from build123d import *

# Parameters (mm, degrees)
F0_W     = 64
F0_H     = 10
F0_R     = 1.75
F1_DEPTH = 4
F2_R     = 2
F3_DEPTH = 10
F4_W     = 64
F4_H     = 9
F5_DEPTH = 6
F6_R     = 1.75
F7_DEPTH = 25
F8_W     = 6
F8_H     = 6
F9_DEPTH = 4
F10_R    = 2


with BuildPart() as f1:
    # F0 (on Front) → F1 (new body)
    with BuildSketch(Plane.XZ):
        Rectangle(F0_W, F0_H)
        with Locations((-27, 0)):
            Circle(F0_R, mode=Mode.SUBTRACT)
        with BuildLine():
            ThreePointArc((28.75, 0), (27, -1.75), (25.25, 0))
            ThreePointArc((25.25, 0), (27, 1.75), (28.75, 0))
        make_face(mode=Mode.SUBTRACT)
    extrude(amount=F1_DEPTH)

    # F2
    f2_edges = [f1.edges().sort_by_distance(p)[0] for p in [
        (-32, -2, 5),
        (32, -2, 5),
    ]]
    fillet(f2_edges, radius=F2_R)

    # F3 (add): a face of the model
    f3_faces = [f1.faces().sort_by_distance(p)[0] for p in [
        (0, -2, -5),
    ]]
    extrude(f3_faces, amount=F3_DEPTH)

    # F4 (on face) → F5 (join)
    with BuildSketch(Plane(origin=(0, 0, 0), x_dir=(-1, 0, 0), z_dir=(0, 1, 0))):
        with Locations((0, -10.5)):
            Rectangle(F4_W, F4_H)
    extrude(amount=F5_DEPTH)

    # F6 (on face) → F7 (cut)
    with BuildSketch(Plane(origin=(0, 6, 0), x_dir=(-1, 0, 0), z_dir=(0, 1, 0))):
        with BuildLine():
            ThreePointArc((-28.75, -10.5), (-27, -12.25), (-25.25, -10.5))
            ThreePointArc((-25.25, -10.5), (-27, -8.75), (-28.75, -10.5))
        make_face()
        with Locations((27, -10.5)):
            Circle(F6_R)
    extrude(amount=-F7_DEPTH, mode=Mode.SUBTRACT)

    # F8 (on face) → F9 (cut)
    with BuildSketch(Plane.XZ.offset(4)):
        with Locations((-27, -10.5)):
            Rectangle(F8_W, F8_H)
        with Locations((27, -10.5)):
            Rectangle(F8_W, F8_H)
    extrude(amount=-F9_DEPTH, mode=Mode.SUBTRACT)

    # F10
    f10_edges = [f1.edges().sort_by_distance(p)[0] for p in [
        (32, 3, -6),
        (-32, 3, -6),
    ]]
    fillet(f10_edges, radius=F10_R)


solid = f1.part
Work out the finished part from the listing and answer in its coordinate system (mm). A direction names the side the tool comes from. Give positions to 0.01 mm unless a question says otherwise; leave off trailing zeros. Loops run counter-clockwise (first coordinate to the right, second up) from the corner with the lowest first, then second, coordinate; pieces in that order, holes last. Notation, with made-up numbers: (-14.5, -11.75) - (40.5, -11.75) arc R20 cw to (40.5, -3.75) - close; hole circle Ø7 at (80.5, 11.25). An arc over 180 degrees is marked (long way). Answer in a Markdown table with one row per item. Add a question column.
Q1. The part is cut by section B-B (x = -27). Determine the outline of the cut face in (y, z).
Q2. Consider line 1 along X through (y, z) = (-0.75, -10); line 2 along Z through (x, y) = (27, 3.5); line 3 along Z through (x, y) = (-27, -2). Determine where each line is inside the solid, lowest interval first.
Q3. Determine the mould class of faces 4 (the cylindrical face through (31.43, 3.04, -6.6)), 5 (the flat face through (-27, -2, -13.5)), 6 (the flat face through (0, 6, -10)), 7 (the flat face through (27, -2, -7.5)) for opening direction Z: released by +Z, released by -Z, zero draft, split by the parting line, or undercut.
Q4. The part is cut by section C-C (y = -0.75). Determine the outline of the cut face in (x, z).
Q5. Each of these flat-tipped pins is pushed along its axis until it touches: P1, Ø1, axis at x = 9.5, z = 2.5, coming from the +Y side; P2, Ø1.8, axis at x = 12.5, y = 3, coming from the +Z side; P3, Ø3, axis at x = 26, z = -10.5, coming from the -Y side; P4, Ø2, axis at x = 27, z = -10.5, coming from the -Y side. Where does it stop, or does it pass through?
Q6. The part is cut by section D-D (y = 5). Determine the outline of the cut face in (x, z), and give its area (3 significant figures).
Q7. The part is cut by section A-A (z = -10.5). Determine the outline of the cut face in (x, y), and give its area (3 significant figures).
Q8. A tool of negligible diameter and unlimited length cuts with its end or side. For faces 1 (the flat face through (0, 3, -6)), 2 (the cylindrical face through (-25.71, 3.04, -9.32)), 3 (the flat face through (24, -2, -11)), from which of +Z, -Z, +X, -X, +Y, -Y can it reach the whole face along a straight path? Write none if from no direction.
Solution:
| question | item | result |
|---|---|---|
| 1 | outline | (-4, -15) - (6, -15) - (6, -12.25) - (0, -12.25) - (0, -13.5) - (-4, -13.5) - close; (-4, -7.5) - (0, -7.5) - (0, -8.75) - (6, -8.75) - (6, -6) - (0, -6) - (0, -1.75) - (-4, -1.75) - close; (-4, 1.75) - (0, 1.75) - (0, 5) - (-4, 5) - close |
| 2 | line 1 | x = -32 to -30, -24 to 24, 30 to 32 |
| 2 | line 2 | z = -15 to -12.25, -8.75 to -6 |
| 2 | line 3 | z = -15 to -13.5, -7.5 to -1.75, 1.75 to 5 |
| 3 | face 4 | released by +Z |
| 3 | face 5 | undercut |
| 3 | face 6 | zero draft |
| 3 | face 7 | undercut |
| 4 | outline | (-32, -15) - (32, -15) - (32, 3) arc R2 ccw to (30, 5) - (-30, 5) arc R2 ccw to (-32, 3) - close; hole (-30, -13.5) - (-24, -13.5) - (-24, -7.5) - (-30, -7.5) - close; hole circle Ø3.5 at (-27, 0); hole (24, -13.5) - (30, -13.5) - (30, -7.5) - (24, -7.5) - close; hole circle Ø3.5 at (27, 0) |
| 5 | P1 | stops at y = 0 |
| 5 | P2 | stops at z = -6 |
| 5 | P3 | stops at y = 0 |
| 5 | P4 | passes through |
| 6 | outline | (-32, -15) - (32, -15) - (32, -8) arc R2 ccw to (30, -6) - (-30, -6) arc R2 ccw to (-32, -8) - close; hole circle Ø3.5 at (-27, -10.5); hole circle Ø3.5 at (27, -10.5) |
| 6 | area | 555 mm² |
| 7 | outline | (-32, -4) - (-30, -4) - (-30, 0) - (-28.75, 0) - (-28.75, 6) - (-32, 6) - close; (-25.25, 0) - (-24, 0) - (-24, -4) - (24, -4) - (24, 0) - (25.25, 0) - (25.25, 6) - (-25.25, 6) - close; (28.75, 0) - (30, 0) - (30, -4) - (32, -4) - (32, 6) - (28.75, 6) - close |
| 7 | area | 550 mm² |
| 8 | face 1 | +Z, +X, -X, +Y |
| 8 | face 2 | +Y, -Y |
| 8 | face 3 | -Y |
